CAD build for the part. Positions are in the model's coordinates, mm. A direction names the side the tool comes from. Coordinates: 2 decimals unless noted, no trailing zeros. Write each loop counter-clockwise with the first axis right and the second up, starting at its lowest first coordinate (ties: lowest second). Pieces come first, ordered by that corner, then holes. Notation, with made-up numbers: M 83.5,58 L 128.5,58 A19 cw 128.5,87 Z; hole C 29,75.25 d4. An arc over 180 degrees is marked long. Answer as CSV lines item,"result". Start each with the question number.
```python
from build123d import *

# Parameters (mm, degrees)
BOSS_EXTRUDE1_DEPTH         = 44.25
BOSS_EXTRUDE2_DEPTH         = 0.85
BOSS_EXTRUDE3_DEPTH         = 1.3
LPATTERN1_COUNT             = 10
LPATTERN1_PITCH             = 9.5
M3_5X0_6_TAPPED_HOLE1_D     = 2.9
M3_5X0_6_TAPPED_HOLE1_DEPTH = 8
M3_5X0_6_TAPPED_HOLE1_TIP   = 0.871247898


with BuildPart() as part:
    # Sketch1 → Boss-Extrude1 (new body, symmetric)
    with BuildSketch(Plane(origin=(0, 0, 0), x_dir=(0, 0, -1), z_dir=(1, 0, 0))):
        Polygon((6.75, 0), (6.75, 2.79), (5.365, 9.1), (-5.365, 9.1), (-6.75, 2.79), (-6.75, 0), align=None)
    extrude(amount=BOSS_EXTRUDE1_DEPTH, both=True)

    # Sketch3 → Boss-Extrude2 (add)
    with BuildSketch(Plane(origin=(44.25, 0, 0), x_dir=(0, 0, -1), z_dir=(1, 0, 0))):
        with BuildLine():
            Line((-6.75, 0), (-7.35, 0))
            Line((-7.35, 0), (-7.35, 18.1))
            ThreePointArc((-7.35, 18.1), (-7.203553391, 18.453553391), (-6.85, 18.6))
            Line((-6.85, 18.6), (6.85, 18.6))
            ThreePointArc((6.85, 18.6), (7.203553391, 18.453553391), (7.35, 18.1))
            Line((7.35, 18.1), (7.35, 0))
            Line((7.35, 0), (6.75, 0))
            Line((6.75, 0), (6.75, 2.79))
            Line((6.75, 2.79), (5.365, 9.1))
            Line((5.365, 9.1), (-5.365, 9.1))
            Line((-5.365, 9.1), (-6.75, 2.79))
            Line((-6.75, 2.79), (-6.75, 0))
        make_face()
    boss_extrude2 = extrude(amount=-BOSS_EXTRUDE2_DEPTH)

    # Mirror1: Boss-Extrude2 across plane
    add(boss_extrude2.mirror(Plane(origin=(0, 0, 0), x_dir=(0, 0, 1), z_dir=(1, 0, 0))))

    # Sketch4 → Boss-Extrude3 (add)
    with BuildSketch(Plane.ZY.offset(-43.4)):
        with BuildLine():
            Line((7.35, 0), (7.35, 12.42))
            Line((7.35, 12.42), (4.588898397, 15.03))
            Line((4.588898397, 15.03), (6.438355915, 16.98652878))
            ThreePointArc((6.438355915, 16.98652878), (6.534203446, 17.527818591), (6.075, 17.83))
            Line((6.075, 17.83), (-6.075, 17.83))
            ThreePointArc((-6.075, 17.83), (-6.534203446, 17.527818591), (-6.438355915, 16.98652878))
            Line((-6.438355915, 16.98652878), (-4.588898397, 15.03))
            Line((-4.588898397, 15.03), (-7.35, 12.42))
            Line((-7.35, 12.42), (-7.35, 0))
            Line((-7.35, 0), (-6.75, 0))
            Line((-6.75, 0), (-6.75, 2.79))
            Line((-6.75, 2.79), (-5.365, 9.1))
            Line((-5.365, 9.1), (5.365, 9.1))
            Line((5.365, 9.1), (6.75, 2.79))
            Line((6.75, 2.79), (6.75, 0))
            Line((6.75, 0), (7.35, 0))
        make_face()
    boss_extrude3 = extrude(amount=BOSS_EXTRUDE3_DEPTH)

    # LPattern1: Boss-Extrude3 ×10
    with Locations(*[(-i * LPATTERN1_PITCH, 0, 0) for i in range(1, LPATTERN1_COUNT)]):
        add(boss_extrude3)

    # M3.5x0.6 Tapped Hole1
    with Locations(Plane(origin=(0, 9.1, 0), x_dir=(1, 0, 0), z_dir=(0, 1, 0))):
        with Locations((-38, 0), (-28.5, 0), (-19, 0), (-9.5, 0), (0, 0), (9.5, 0), (19, 0), (28.5, 0), (38, 0)):
            Hole(M3_5X0_6_TAPPED_HOLE1_D / 2, depth=M3_5X0_6_TAPPED_HOLE1_DEPTH)
            with Locations((0, 0, -(M3_5X0_6_TAPPED_HOLE1_DEPTH + M3_5X0_6_TAPPED_HOLE1_TIP / 2))):  # 118° drill point
                Cone(0, M3_5X0_6_TAPPED_HOLE1_D / 2, M3_5X0_6_TAPPED_HOLE1_TIP, mode=Mode.SUBTRACT)


solid = part.part
```
1) Two-plate mould, pull along Y, no slides. Class faces 1 (the flat face through (-23.741, 13.743, -5.95)), 2 (the flat face through (38.057, 5.901, -6.067)), 3 (the flat face through (-38, 1, -6.75)): pulls with the +Y half, pulls with the -Y half, needs draft (parallel to the pull), parting line crosses it, or undercut.
2) Pin check, flat tips, straight feed: P1, Ø3, axis at x = -37.5, y = 2, coming from the -Z side; P2, Ø8, axis at x = 0, y = 5, coming from the +Z side; P3, Ø5, axis at x = 10, z = 2.5, coming from the -Y side; P4, Ø4.5, axis at x = 38, z = 0, coming from the +Y side. Stop position of each tip, or through.
3) Band-saw the part on A-A, the plane x = 35. List the corners of the cut face in (y, z) (3 decimals), plus the area to 3 significant figures.
4) Probe L1, parallel to Y at x = -26.5, z = 2.5; L2, parallel to X at y = 16.25, z = 6.5; L3, parallel to Z at x = 38, y = 6. List the from-to ranges inside material, lowest first. Write a range as [from, to].
5) Tool access for faces 4 (the flat face through (28.557, 5.989, 6.048)), 5 (the flat face through (-43.4, 18, 0)), 6 (the flat face through (-37.943, 5.901, -6.067)): list every direction of +Z, -Z, +X, -X, +Y, -Y with a clear straight run to the whole face (end or side of a thin tool).
6) Band-saw the part on B-B, the plane y = 5.25. State how many separate pieces and enclosed holes the cut face has, plus the area to 3 significant figures.
Result sheet:
1,face 1,"undercut"
1,face 2,"pulls with the +Y half"
1,face 3,"needs draft"
2,P1,"stops at z = -6.75"
2,P2,"stops at z = 6.75"
2,P3,"stops at y = 0"
2,P4,"stops at y = 9.1"
3,outline,"M 0,-6.75 L 2.79,-6.75 L 9.1,-5.365 L 9.1,5.365 L 2.79,6.75 L 0,6.75 Z"
3,area,"114 mm²"
4,L1,"y = [0, 9.1]"
4,L2,"x = [-44.25, -43.4], [43.4, 44.25]"
4,L3,"z = [-6.05, -1.45], [1.45, 6.05]"
5,face 4,"+Z, +Y"
5,face 5,"none"
5,face 6,"-Z, +Y"
6,separate pieces,"1"
6,enclosed holes,"9"
6,area,"1,070 mm²"
